```python
from build123d import *

# Parameters (mm, degrees)
F0_W     = 508
F0_H     = 254
F1_DEPTH = 50.8
F2_W     = 457.2
F2_H     = 203.2
F3_DEPTH = 40.64
F4_W     = 457.2
F4_H     = 50.8
F5_DEPTH = 10.16


with BuildPart() as f1:
    # F0 (on Top) → F1 (new body)
    with BuildSketch(Plane.XY):
        Rectangle(F0_W, F0_H)
    extrude(amount=-F1_DEPTH)

    # F2 (on face) → F3 (cut)
    with BuildSketch(Plane(origin=(0, 0, -50.8), x_dir=(1, 0, 0), z_dir=(0, 0, -1))):
        Rectangle(F2_W, F2_H)
    extrude(amount=-F3_DEPTH, mode=Mode.SUBTRACT)

    # F4 (on face) → F5 (cut)
    with BuildSketch(Plane.XY):
        with Locations((-25.4, 0)):
            Rectangle(F4_W, F4_H)
    extrude(amount=-F5_DEPTH, mode=Mode.SUBTRACT)


solid = f1.part
```
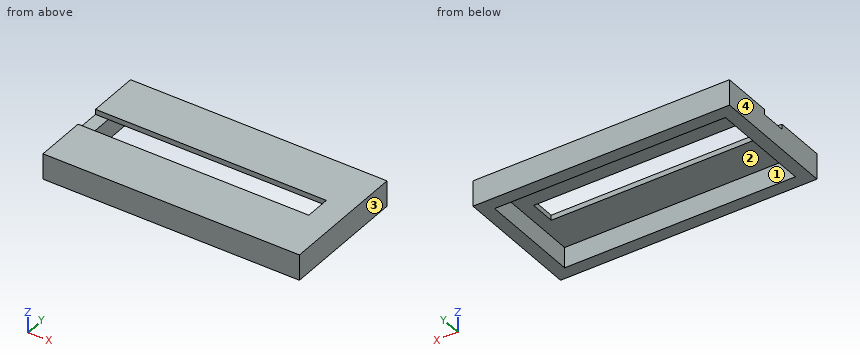
Input: part model. Units: mm. Frame: model coordinates. Face numbers are marked on the shaded views. Coordinates: 2 decimals unless noted, no trailing zeros. Write each loop counter-clockwise with the first axis right and the second up, starting at its lowest first coordinate (ties: lowest second). Pieces come first, ordered by that corner, then holes. Notation, with made-up numbers: (33, 80) - (53, 80) arc R18 cw to (53, 84) - close; hole circle Ø8 at (40.25, -32). An arc over 180 degrees is marked (long way). Put each result on its own line as item: value. Start each with the question number.
1) Cut plane C-C (z = -36). Return the cut outline in (x, y).
2) Ray query, L1, parallel to Y at x = 113, z = -9; L2, parallel to Y at x = 120, z = -30.5; L3, parallel to X at y = -30, z = -34. Return the intervals inside material, ascending.
3) Cut plane A-A (x = 168.5). Return the cut outline in (y, z).
4) Cut plane D-D (x = 220). Return the cut outline in (y, z), plus the area to 3 significant figures.
5) Mould query, pull axis X, two halves, no side actions, for the marked faces 1, 2, 3 and 4. Classes: pulls with the +X half, pulls with the -X half, needs draft (parallel to the pull), parting line crosses it, or undercut.
6) Cut plane B-B (y = 0.5). Return the cut outline in (x, z).
7) Contact query for flat-ended pins moving along their axis: pin 1 (2 mm diameter, centred on x = -158, y = 29.5, fed in from +Z); pin 2 (5 mm diameter, centred on y = 9, z = -5.5, fed in from -X); pin 3 (2 mm diameter, centred on x = 101, y = 58, fed in from -Z). Output: stop coordinate, or through.
Resolved:
1. outline: (-254, -127) - (254, -127) - (254, 127) - (-254, 127) - close; hole (-228.6, -101.6) - (228.6, -101.6) - (228.6, 101.6) - (-228.6, 101.6) - close
2. L1: y = -127 to -25.4, 25.4 to 127
2. L2: y = -127 to -101.6, 101.6 to 127
2. L3: x = -254 to -228.6, 228.6 to 254
3. outline: (-127, -50.8) - (-101.6, -50.8) - (-101.6, -10.16) - (-25.4, -10.16) - (-25.4, 0) - (-127, 0) - close; (25.4, -10.16) - (101.6, -10.16) - (101.6, -50.8) - (127, -50.8) - (127, 0) - (25.4, 0) - close
4. outline: (-127, -50.8) - (-101.6, -50.8) - (-101.6, -10.16) - (101.6, -10.16) - (101.6, -50.8) - (127, -50.8) - (127, 0) - (-127, 0) - close
4. area: 4,650 mm2
5. face 1: undercut
5. face 2: undercut
5. face 3: pulls with the +X half
5. face 4: pulls with the -X half
6. outline: (-254, -50.8) - (-228.6, -50.8) - (-228.6, -10.16) - (-254, -10.16) - close; (203.2, -10.16) - (228.6, -10.16) - (228.6, -50.8) - (254, -50.8) - (254, 0) - (203.2, 0) - close
7. pin 1: stops at z = 0
7. pin 2: stops at x = 203.2
7. pin 3: stops at z = -10.16
